Read the model definition and answer for the solid it produces. Units are mm, in the model's axes. A direction names the side the tool comes from. Coordinates: 2 decimals unless noted, no trailing zeros. Write each loop counter-clockwise with the first axis right and the second up, starting at its lowest first coordinate (ties: lowest second). Pieces come first, ordered by that corner, then holes. Notation, with made-up numbers: (22, 67.5) -> (76, 67.5) arc R33 cw to (76, 106.5) -> close; hole circle Ø1 at (53.5, 79). An arc over 180 degrees is marked (long way). One line per item, written item: value. Start each with the question number.
1. Find section A-A, the plane x = 9. Write down the section's boundary in (y, z), and give its area (3 significant figures).
2. Find section C-C, the plane z = -1.25. State how many separate pieces and enclosed holes the cut face has, and give its area (3 significant figures).
3. For faces 3 (the cylindrical face through (30.432, 5.406, -8.698)), 4 (the flat face through (17, 27.15, -2)), 5 (the cylindrical face through (18.574, 47.465, -0.996)), determine the directions among +Z, -Z, +X, -X, +Y, -Y from which every point of the face is accessible in a straight line to the end or side of a thin tool.
4. Consider line 1 along X through (y, z) = (46, -0.5); line 2 along X through (y, z) = (24, -10.5); line 3 along Y through (x, z) = (5, -6.5). Determine where each line is inside the solid, lowest interval first.
5. Find section B-B, the plane y = 38. Write down the section's boundary in (x, z).
6. Given P1, Ø3, axis at x = 5.5, z = -1.5, coming from the +Y side; P2, Ø4, axis at x = 8, y = 40.5, coming from the +Z side; P3, Ø1.1, axis at x = 28.5, z = -1, coming from the +Y side; P4, Ø1.7, axis at x = 17, y = 4.5, coming from the +Z side, each flat-ended and moving along its own axis, determine where each tip first touches the part or whether it passes through.
7. For a pull along X with two mould halves and no side action, classify faces 1 (the flat face through (16.8, 49.8, -12.5)), 2 (the flat face through (14.54, 7.44, -2.46)) as pulls with the +X half, pulls with the -X half, needs draft (parallel to the pull), parting line crosses it, or undercut.
8. Find section D-D, the plane y = 11.5. Write down the section's boundary in (x, z).
```python
from build123d import *

# Parameters (mm, degrees)
SKETCH_1_W          = 12.5
SKETCH_1_H          = 50
EXTRUDE_1_DEPTH     = 34
SKETCH_2_R          = 7.5
CUT_EXTRUDE_1_DEPTH = 13.25
SKETCH_3_R          = 1.55
SKETCH_3_R_2        = 1.65
CUT_EXTRUDE_2_DEPTH = 13.5
CUT_EXTRUDE_3_DEPTH = 5
SKETCH_5_R          = 5.5
CUT_EXTRUDE_4_DEPTH = 35
EXTRUDE_2_DEPTH     = 17
SKETCH_7_R          = 1.65
CUT_EXTRUDE_5_DEPTH = 6
CUT_EXTRUDE_6_DEPTH = 9


with BuildPart() as part:
    # 草图1 → 凸台-拉伸1 (new body)
    with BuildSketch(Plane(origin=(0, 0, 0), x_dir=(0, 0, -1), z_dir=(1, 0, 0))):
        with Locations((6.25, 25)):
            Rectangle(SKETCH_1_W, SKETCH_1_H)
    extrude(amount=EXTRUDE_1_DEPTH)

    # 草图2 → 切除-拉伸1 (cut, symmetric)
    with BuildSketch(Plane.ZY.offset(-17)):
        with Locations((-12.5, 18)):
            Circle(SKETCH_2_R)
        with Locations((-12.5, 42)):
            Circle(SKETCH_2_R)
    extrude(amount=CUT_EXTRUDE_1_DEPTH, both=True, mode=Mode.SUBTRACT)

    # 草图3 → 切除-拉伸2 (cut, through all)
    with BuildSketch(Plane.XY):
        with Locations((29, 30)):
            Circle(SKETCH_3_R)
        with Locations((5, 30)):
            Circle(SKETCH_3_R_2)
        with Locations((17, 30)):
            Circle(SKETCH_3_R)
        with Locations((5, 6)):
            Circle(SKETCH_3_R_2)
        with Locations((17, 6)):
            Circle(SKETCH_3_R)
        with Locations((29, 6)):
            Circle(SKETCH_3_R)
    extrude(amount=-CUT_EXTRUDE_2_DEPTH, mode=Mode.SUBTRACT)

    # 草图4 → 切除-拉伸3 (cut)
    with BuildSketch(Plane.XY):
        Polygon((18.645448267, 27.15), (20.290896534, 30), (18.645448267, 32.85), (15.354551733, 32.85), (13.709103466, 30), (15.354551733, 27.15), align=None)
        Polygon((18.645448267, 3.15), (20.290896534, 6), (18.645448267, 8.85), (15.354551733, 8.85), (13.709103466, 6), (15.354551733, 3.15), align=None)
        Polygon((30.645448267, 3.15), (32.290896534, 6), (30.645448267, 8.85), (27.354551733, 8.85), (25.709103466, 6), (27.354551733, 3.15), align=None)
        Polygon((6.645448267, 3.15), (8.290896534, 6), (6.645448267, 8.85), (3.354551733, 8.85), (1.709103466, 6), (3.354551733, 3.15), align=None)
    extrude(amount=-CUT_EXTRUDE_3_DEPTH, mode=Mode.SUBTRACT)

    # 草图5 → 切除-拉伸4 (cut, through all)
    with BuildSketch(Plane(origin=(34, 0, 0), x_dir=(0, 0, -1), z_dir=(1, 0, 0))):
        with Locations((12.5, 18)):
            Circle(SKETCH_5_R)
        with Locations((12.5, 42)):
            Circle(SKETCH_5_R)
    extrude(amount=-CUT_EXTRUDE_4_DEPTH, mode=Mode.SUBTRACT)

    # 草图6 → 凸台-拉伸2 (add, symmetric)
    with BuildSketch(Plane.ZY.offset(-17)):
        Polygon((0, 50), (5, 50), (5, 45), (0, 40), align=None)
    extrude(amount=EXTRUDE_2_DEPTH, both=True)

    # 草图7 → 切除-拉伸5 (cut, through all)
    with BuildSketch(Plane(origin=(0, 45, 0), x_dir=(1, 0, 0), z_dir=(0, 1, 0))):
        with Locations((5, 0.5)):
            Circle(SKETCH_7_R)
        with Locations((17, 0.5)):
            Circle(SKETCH_7_R)
        with Locations((29, 0.5)):
            Circle(SKETCH_7_R)
    extrude(amount=CUT_EXTRUDE_5_DEPTH, mode=Mode.SUBTRACT)

    # 草图8 → 切除-拉伸6 (cut)
    with BuildSketch(Plane(origin=(0, 45, 0), x_dir=(1, 0, 0), z_dir=(0, 1, 0))):
        Polygon((7.85, -0.590838694), (7.85, 2.145448267), (5, 3.790896534), (2.15, 2.145448267), (2.15, -0.481963635), (2.15, -5), (7.85, -5), align=None)
        Polygon((19.85, -0.590838694), (19.85, 2.145448267), (17, 3.790896534), (14.15, 2.145448267), (14.15, -0.481963635), (14.15, -5), (19.85, -5), align=None)
        Polygon((31.85, -0.590838694), (31.85, 2.145448267), (29, 3.790896534), (26.15, 2.145448267), (26.15, -0.481963635), (26.15, -5), (31.85, -5), align=None)
    extrude(amount=-CUT_EXTRUDE_6_DEPTH, mode=Mode.SUBTRACT)


solid = part.part
```
Answer block:
1. outline: (0, -12.5) -> (10.5, -12.5) arc R7.5 cw to (25.5, -12.5) -> (34.5, -12.5) arc R7.5 cw to (49.5, -12.5) -> (50, -12.5) -> (50, 5) -> (45, 5) -> (40, 0) -> (0, 0) -> close
1. area: 486 mm2
2. separate pieces: 1
2. enclosed holes: 6
2. area: 1,370 mm2
3. face 3: +Z, -Z
3. face 4: +Z
3. face 5: +Y
4. line 1: x = 0 to 3.35, 6.65 to 15.35, 18.65 to 27.35, 30.65 to 34
4. line 2: x = 0 to 3.75, 30.25 to 34
4. line 3: y = 0 to 4.35, 7.65 to 13.5, 22.5 to 28.35, 31.65 to 37.5, 46.5 to 50
5. outline: (0, -8.73) -> (3.75, -8.73) -> (3.75, -6.16) -> (30.25, -6.16) -> (30.25, -8.73) -> (34, -8.73) -> (34, 0) -> (31.85, 0) -> (31.85, -2.15) -> (29, -3.79) -> (26.15, -2.15) -> (26.15, 0) -> (19.85, 0) -> (19.85, -2.15) -> (17, -3.79) -> (14.15, -2.15) -> (14.15, 0) -> (7.85, 0) -> (7.85, -2.15) -> (5, -3.79) -> (2.15, -2.15) -> (2.15, 0) -> (0, 0) -> close
6. P1: stops at y = 50
6. P2: stops at z = 2.5
6. P3: stops at y = 36
6. P4: stops at z = -5
7. face 1: needs draft
7. face 2: undercut
8. outline: (0, -12.5) -> (3.75, -12.5) -> (3.75, -8.76) -> (30.25, -8.76) -> (30.25, -12.5) -> (34, -12.5) -> (34, 0) -> (0, 0) -> close
